The model under review builds one solid part; all positions refer to its coordinate system, in mm. A direction names the side the tool comes from. Round coordinates to 2 decimals unless told otherwise and drop trailing zeros. Write each loop counter-clockwise with the first axis right and the second up, starting at its lowest first coordinate (ties: lowest second). Pieces come first, ordered by that corner, then holes.
Item 1: Machinability: for faces 1 (the face through (7.199, 5.479, 4.535)), 2 (the face through (0, 2, 4.25)), 3 (the face through (0, 0, 0)), 4 (the face through (0, 6, 4.25)), 5 (the face through (-7.215, 5.479, 4.551)), which of the approach directions +Z, -Z, +X, -X, +Y, -Y give a long, thin tool a straight path to every point of the face, cutting with its end or side? Answer none if there is none.
Item 2: Add section B-B (x = -5). Give the boundary of the cut face in (y, z).
Item 3: Draft analysis for pull direction X (two halves, no side actions). For faces 6 (the face through (0, 4, 1)), 7 (the face through (-7.215, 3.549, 5.949)), 8 (the face through (0.17, 3.29, -1.07)), state which applies: +X half, -X half, draft (parallel to the pull), parting line (faces both ways), or undercut.
Item 4: Add section D-D (z = -1.5). Give the boundary of the cut face in (x, y), plus the area to 3 significant figures.
Item 5: To check wall thickness, follow L1, parallel to Z at x = 1.75, y = 5.5; L2, parallel to Y at x = 0, z = -3.25; L3, parallel to Y at x = 0, z = -0.75. State the ranges of each line that lie inside material, in increasing order.
Item 6: Clearance check with a flat-ended pin moving along its axis: pin 1 Ø4 at (x, z) = (2.5, 1.5) entering from +Y. State where the tip first meets the part, or that it passes through.
Item 7: Add section C-C (y = 2). Give the boundary of the cut face in (x, z).
```python
from build123d import *

# Parameters (mm, degrees)
SKETCH1_W           = 15
SKETCH1_H           = 12.5
BOSS_EXTRUDE1_DEPTH = 7
SKETCH2_W           = 15
SKETCH2_H           = 6.5
CUT_EXTRUDE2_DEPTH  = 3
SKETCH3_R           = 1.3
CUT_EXTRUDE3_DEPTH  = 10.5
FILLET1_R           = 1


with BuildPart() as part:
    # Sketch1 → Boss-Extrude1 (new body)
    with BuildSketch(Plane(origin=(0, 0, 0), x_dir=(1, 0, 0), z_dir=(0, 1, 0))):
        Rectangle(SKETCH1_W, SKETCH1_H)
    extrude(amount=BOSS_EXTRUDE1_DEPTH)

    # Sketch2 → Cut-Extrude2 (cut)
    with BuildSketch(Plane(origin=(0, 7, 0), x_dir=(1, 0, 0), z_dir=(0, 1, 0))):
        with Locations((0, -1)):
            Rectangle(SKETCH2_W, SKETCH2_H)
    extrude(amount=-CUT_EXTRUDE2_DEPTH, mode=Mode.SUBTRACT)

    # Sketch3 → Cut-Extrude3 (cut)
    with BuildSketch(Plane(origin=(0, 0, -6.25), x_dir=(-1, 0, 0), z_dir=(0, 0, -1))):
        with Locations((0, 2)):
            Circle(SKETCH3_R)
    extrude(amount=-CUT_EXTRUDE3_DEPTH, mode=Mode.SUBTRACT)

    # Fillet1
    fillet1_edges = [part.edges().sort_by_distance(p)[0] for p in [
        (7.5, 5.5, -2.25),
        (7.5, 5.5, 4.25),
        (-7.5, 5.5, 4.25),
        (-7.5, 5.5, -2.25),
        (7.5, 3.5, 6.25),
        (-7.5, 3.5, 6.25),
        (-7.5, 3.5, -6.25),
        (7.5, 3.5, -6.25),
    ]]
    fillet(fillet1_edges, radius=FILLET1_R - 0.0001)  # a hair under: the kernel refuses the full size


solid = part.part
```
Numbers:
1. face 1: +X, +Y
1. face 2: -Z
1. face 3: +Z, -Z, +X, -X, -Y
1. face 4: +X, -X, +Y
1. face 5: -X, +Y
2. outline: (0, -6.25) - (7, -6.25) - (7, -2.25) - (4, -2.25) - (4, 4.25) - (7, 4.25) - (7, 6.25) - (0, 6.25) - close
3. face 6: draft
3. face 7: -X half
3. face 8: undercut
4. outline: (-7.5, 0) - (7.5, 0) - (7.5, 4) - (-7.5, 4) - close; hole circle Ø2.6 at (0, 2)
4. area: 54.7 mm2
5. L1: z = -6.25 to -2.25, 4.25 to 6.25
5. L2: y = 0 to 0.7, 3.3 to 7
5. L3: y = 0 to 0.7, 3.3 to 4
6. pin 1: stops at y = 4
7. outline: (-7.5, -5.25) arc R1 ccw to (-6.5, -6.25) - (-1.3, -6.25) - (-1.3, 4.25) - (1.3, 4.25) - (1.3, -6.25) - (6.5, -6.25) arc R1 ccw to (7.5, -5.25) - (7.5, 5.25) arc R1 ccw to (6.5, 6.25) - (-6.5, 6.25) arc R1 ccw to (-7.5, 5.25) - close
